from build123d import *

# Parameters (mm, degrees)
CUT_EXTRUDE1_DEPTH = 0.762
CHAMFER1_SIZE      = 0.508
CHAMFER1_SIZE2     = 1.89588181


with BuildPart() as part:
    # Sketch1 → Revolve1 (revolve)
    with BuildSketch(Plane(origin=(0, 0, 0), x_dir=(0, 0, -1), z_dir=(1, 0, 0))):
        with BuildLine():
            Line((0, 0), (-6.35, 0))
            Line((-6.35, 0), (-6.35, 1.016))
            Line((-6.35, 1.016), (-1.016, 1.016))
            Line((-1.016, 1.016), (-1.016, 1.778))
            Line((-1.016, 1.778), (-0.762, 1.778))
            ThreePointArc((-0.762, 1.778), (-0.223184633, 1.554815367), (0, 1.016))
            Line((0, 1.016), (0, 0))
        make_face()
    revolve(axis=Axis((0, 0, 0), (0, 0, 1)))

    # Sketch2 → Cut-Extrude1 (cut)
    with BuildSketch(Plane(origin=(0, 0, 0), x_dir=(-1, 0, 0), z_dir=(0, 0, -1))):
        Polygon((0.195962003, -1.459943378), (-0.195962003, -1.459943378), (-0.195962003, -0.348829462), (-0.348829462, -0.195962003), (-1.459943378, -0.195962003), (-1.459943378, 0.195962003), (-0.348829462, 0.195962003), (-0.195962003, 0.348829462), (-0.195962003, 1.459943378), (0.195962003, 1.459943378), (0.195962003, 0.348829462), (0.348829462, 0.195962003), (1.459943378, 0.195962003), (1.459943378, -0.195962003), (0.348829462, -0.195962003), (0.195962003, -0.348829462), align=None)
    extrude(amount=-CUT_EXTRUDE1_DEPTH, mode=Mode.SUBTRACT)

    # Chamfer1
    chamfer1_edges = [part.edges().sort_by_distance(p)[0] for p in [
        (0, -1.016, 6.35),
    ]]
    chamfer1_side = [part.faces().sort_by_distance(p)[0] for p in [
        (0, 0, 6.35),
    ]]
    chamfer(chamfer1_edges, length=CHAMFER1_SIZE, length2=CHAMFER1_SIZE2, reference=chamfer1_side[0])


solid = part.part
Verification items for the finished model (mm, model axes). A direction names the side the tool comes from. Round coordinates to 2 decimals unless told otherwise and drop trailing zeros. Loops run counter-clockwise (first coordinate to the right, second up) from the corner with the lowest first, then second, coordinate; pieces in that order, holes last. Notation, with made-up numbers: (26.25, 89) - (76.25, 89) arc R24 cw to (76.25, 112) - close; hole circle Ø1 at (54, -7.5). An arc over 180 degrees is marked (long way). Use one line per item in the form item = value.
1. Scan lines: probe 1 along Z at (x, y) = (-0.25, 0.05); probe 2 along X at (y, z) = (-0.4, 3); probe 3 along Z at (x, y) = (-0.55, 1.6). Record each from-to range of solid material in increasing order.
A:
probe_1 = 0.76 to 6.35
probe_2 = -0.93 to 0.93
probe_3 = 0.41 to 1.02
2. Section check A-A on y = 0. Record the cut outline in (x, z), and give its area (3 significant figures).
A:
outline = (-1.78, 0.76) arc R0.76 ccw to (-1.46, 0.14) - (-1.46, 0.76) - (1.46, 0.76) - (1.46, 0.14) arc R0.76 ccw to (1.78, 0.76) - (1.78, 1.02) - (1.02, 1.02) - (1.02, 4.45) - (0.51, 6.35) - (-0.51, 6.35) - (-1.02, 4.45) - (-1.02, 1.02) - (-1.78, 1.02) - close
area = 11.1 mm²
3. Section check C-C on z = 1.25. Record the cut outline in (x, y), and give its area (3 significant figures).
A:
outline = circle Ø2.03 at (0, 0)
area = 3.24 mm²
4. Gauge pin test, flat ends, axial feed: pin 1 Ø0.8 at (y, z) = (1, 0.5) entering from -X; pin 2 Ø0.6 at (x, z) = (1, 0.5) entering from +Y; pin 3 Ø0.8 at (x, z) = (1, 0.5) entering from -Y. Record the tip position at first contact, or that the pin passes through.
A:
pin_1 = -1.65
pin_2 = 1.61
pin_3 = -1.65
5. Draft check along X on faces 1 (the flat face through (0, 0, 0.762)), 2 (the conical face through (0.431, -0.563, 5.599)), 3 (the flat face through (0, 0, 6.35)). Enter one of: pulls with the +X half, pulls with the -X half, needs draft (parallel to the pull), parting line crosses it, or undercut.
A:
face_1 = undercut
face_2 = parting line crosses it
face_3 = needs draft
6. Access from +Z, -Z, +X, -X, +Y, -Y to the whole of each face (thin tool, end or side, straight path). Record for faces 4 (the flat face through (0.5, -0.5, 0)), 5 (the cylindrical face through (0.99, -0.22, 2.71)).
A:
face_4 = -Z, +X, -X, +Y, -Y
face_5 = +Z
